Design review of the part built by this model. Coordinates are the model's own, in mm. Coordinates: 2 decimals unless noted, no trailing zeros. Loops run counter-clockwise (first coordinate to the right, second up) from the corner with the lowest first, then second, coordinate; pieces in that order, holes last. Notation, with made-up numbers: M -4,-1 L 15,-1 A15 ccw 15,24 Z; hole C 80,26.25 d1. An arc over 180 degrees is marked long. Answer as a JSON object with one key per item and string values. Group by question number.
1. To check wall thickness, follow probe 1 along X at (y, z) = (-43, 3); probe 2 along Y at (x, z) = (-58, 2.35); probe 3 along Y at (x, z) = (-25, 2.1). State the ranges of each line that lie inside material, in increasing order.
2. Consider section D-D (y = -105). State the section outline as (x, z) points, then the cut area to 3 significant figures.
3. Insertion check: pin 1 (5 mm diameter, centred on x = -110.5, y = -43.5, fed in from +Z); pin 2 (2 mm diameter, centred on x = -104, y = -80, fed in from -Z); pin 3 (2.5 mm diameter, centred on y = -125, z = 7, fed in from +X); pin 4 (2.5 mm diameter, centred on y = -13.5, z = 8.5, fed in from +X). Each pin has a flat end and moves straight along its axis. Give the tip position at first contact, or say it passes through.
4. Consider section C-C (x = -119). State the section outline as (y, z) points.
5. Consider section A-A (x = -100). State the section outline as (y, z) points, then the cut area to 3 significant figures.
6. Consider section B-B (z = 8.5). State the section outline as (x, y) points, then the cut area to 3 significant figures.
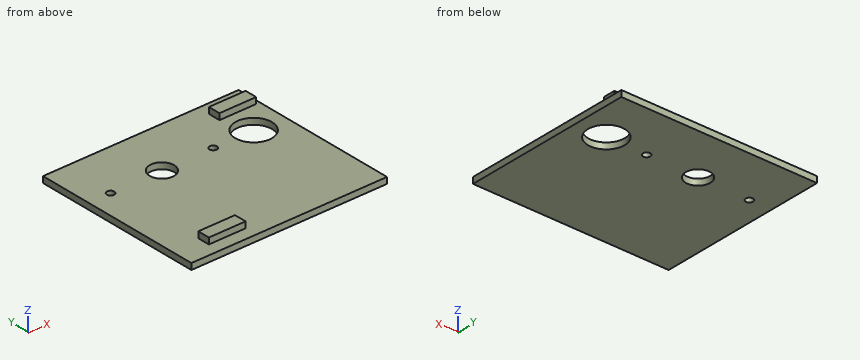
from build123d import *

# Parameters (mm, degrees)
SKETCH1_W           = 160
SKETCH1_H           = 140
BOSS_EXTRUDE1_DEPTH = 5
SKETCH2_W           = 30
SKETCH2_H           = 10
BOSS_EXTRUDE2_DEPTH = 5
SKETCH4_R           = 3
SKETCH4_R_2         = 10
SKETCH4_R_3         = 15
CUT_EXTRUDE1_DEPTH  = 15


with BuildPart() as part:
    # Sketch1 → Boss-Extrude1 (new body)
    with BuildSketch(Plane.XY):
        with Locations((-80, -70)):
            Rectangle(SKETCH1_W, SKETCH1_H)
    extrude(amount=BOSS_EXTRUDE1_DEPTH)

    # Sketch2 → Boss-Extrude2 (add)
    with BuildSketch(Plane.XY.offset(5)):
        with Locations((-18, -15)):
            Rectangle(SKETCH2_W, SKETCH2_H)
        with Locations((-122, -125)):
            Rectangle(SKETCH2_W, SKETCH2_H)
    extrude(amount=BOSS_EXTRUDE2_DEPTH)

    # Sketch4 → Cut-Extrude1 (cut)
    with BuildSketch(Plane.XY.offset(10)):
        with Locations(Location((-142, -43, 0), (0, 0, 180))):
            Circle(SKETCH4_R)
        with Locations(Location((-100, -43, 0), (0, 0, 180))):
            Circle(SKETCH4_R_2)
        with Locations(Location((-58, -43, 0), (0, 0, 180))):
            Circle(SKETCH4_R)
        with Locations(Location((-25, -43, 0), (0, 0, 180))):
            Circle(SKETCH4_R_3)
    extrude(amount=-CUT_EXTRUDE1_DEPTH, mode=Mode.SUBTRACT)


solid = part.part
Findings below:
{
 "1": {"probe 1": "x = -160 to -145, -139 to -110, -90 to -61, -55 to -40, -10 to 0", "probe 2": "y = -140 to -46, -40 to 0", "probe 3": "y = -140 to -58, -28 to 0"},
 "2": {"outline": "M -160,0 L 0,0 L 0,5 L -160,5 Z", "area": "800 mm^2"},
 "3": {"pin 1": "stops at z = 5", "pin 2": "stops at z = 0", "pin 3": "stops at x = -107", "pin 4": "stops at x = -3"},
 "4": {"outline": "M -140,0 L 0,0 L 0,5 L -120,5 L -120,10 L -130,10 L -130,5 L -140,5 Z"},
 "5": {"outline": "M -140,0 L -53,0 L -53,5 L -140,5 Z; M -33,0 L 0,0 L 0,5 L -33,5 Z", "area": "600 mm^2"},
 "6": {"outline": "M -137,-130 L -107,-130 L -107,-120 L -137,-120 Z; M -33,-20 L -3,-20 L -3,-10 L -33,-10 Z", "area": "600 mm^2"}
}
